Check sheet for the modelled part. Datum: model origin and axes. Units: mm. Face numbers are marked on the shaded views. Give positions to 0.01 mm unless a question says otherwise; leave off trailing zeros. Loops run counter-clockwise (first coordinate to the right, second up) from the corner with the lowest first, then second, coordinate; pieces in that order, holes last. Notation, with made-up numbers: (64, 12.25) - (85, 12.25) arc R18 ccw to (85, 42.25) - close; hole circle Ø9 at (29.25, 64.5). An arc over 180 degrees is marked (long way). Use CSV: the item, a comma, the result in double quotes.
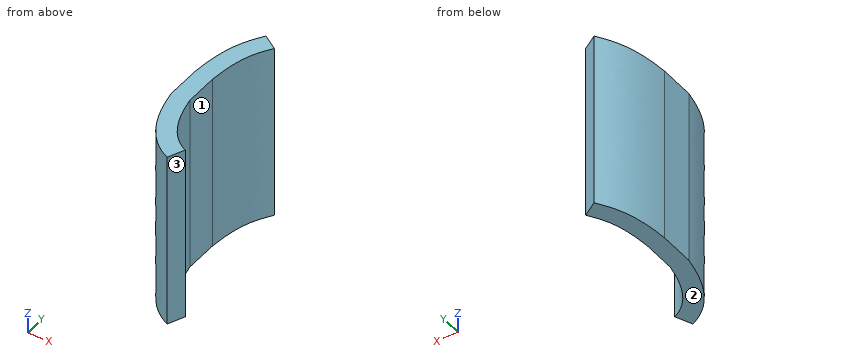
from build123d import *

# Parameters (mm, degrees)
BOSS_EXTRUDE1_DEPTH = 100


with BuildPart() as part:
    # Sketch2 → Boss-Extrude1 (new body)
    with BuildSketch(Plane.XY):
        with BuildLine():
            add(Edge.make_bspline(
                [(0, 10), (1.533515377, 33.319151282), (7.303166768, 41.847313143), (12.598069813, 50)],
                knots=[0, 0, 0, 0, 1, 1, 1, 1], degree=3))
            Line((0, 10), (0, 0))
            Line((0, 0), (0, -10))
            add(Edge.make_bspline(
                [(0, -10), (5.162408831, -41.387474282), (24.940857621, -50)],
                knots=[0, 0, 0, 1, 1, 1], degree=2))
            Line((24.940857621, -50), (28.933264328, -40.831538368))
            add(Edge.make_bspline(
                [(10, -9.163474156), (10.056385248, -9.489994067), (10.218691454, -10.40274145), (10.608632812, -12.423582905), (11.217159707, -15.147367418), (12.036197112, -18.205876092), (13.241421003, -22.010184853), (14.946624948, -26.249584187), (17.264049235, -30.529570228), (19.809393711, -34.048772515), (22.561889728, -36.886540275), (25.055614435, -38.769105307), (27.20346958, -40.024321521), (28.35268275, -40.578724115), (28.933264328, -40.831538368)],
                knots=[0.013914319, 0.013914319, 0.013914319, 0.013914319, 0.03125, 0.0625, 0.125, 0.1875, 0.25, 0.375, 0.5, 0.625, 0.75, 0.875, 0.9375, 1, 1, 1, 1], degree=3))
            Line((10, -9.163474156), (10, 0))
            Line((10, 0), (10, 9.66613227))
            add(Edge.make_bspline(
                [(10, 9.66613227), (10.044832415, 10.325668243), (10.145323413, 11.665207775), (10.370656318, 14.172612644), (10.703199446, 17.109625288), (11.171932341, 20.302311995), (11.878481202, 24.159772501), (12.891303178, 28.284538206), (14.25087497, 32.33124201), (15.719533079, 35.71915175), (17.301714969, 38.710204086), (18.75029356, 41.091588426), (19.993631129, 43.030159771), (20.657608588, 44.049863049), (20.984546989, 44.553257801)],
                knots=[0.004937345, 0.004937345, 0.004937345, 0.004937345, 0.036033053, 0.067128761, 0.129320177, 0.191511593, 0.253703009, 0.378085841, 0.502468673, 0.626851505, 0.751234336, 0.875617168, 0.937808584, 1, 1, 1, 1], degree=3))
            Line((20.984546989, 44.553257801), (12.598069813, 50))
        make_face()
    extrude(amount=BOSS_EXTRUDE1_DEPTH)


solid = part.part
1. Sectioned sample at A-A, the plane y = 3. Record the boundary of the cut face in (x, z), and give its area (3 significant figures).
Completed:
outline,"(0, 0) - (10, 0) - (10, 100) - (0, 100) - close"
area,"1,000 mm²"
2. Release check for a two-part mould opening along Y. For the marked faces 1, 2 and 3 record: released by +Y, released by -Y, zero draft, split by the parting line, or undercut.
Completed:
face 1,"undercut"
face 2,"zero draft"
face 3,"released by -Y"
3. Go/stop test with flat-tipped pins: pin 1 Ø6 at (x, z) = (19.5, 72) entering from -Y; pin 2 Ø1.5 at (x, z) = (8.5, 15.5) entering from +Y; pin 3 Ø6 at (x, y) = (21, -28.5) entering from -Z; pin 4 Ø4 at (y, z) = (-38.5, 21.5) entering from +X. Record where each tip stops, or that it passes through.
Completed:
pin 1,"stops at y = -48.82"
pin 2,"stops at y = 44.69"
pin 3,"passes through"
pin 4,"stops at x = 28.2"
4. Scan lines: line 1 along Y through (x, z) = (20.25, 66); line 2 along X through (y, z) = (-8, 16); line 3 along Y through (x, z) = (6.25, 16). Record each from-to range of solid material in increasing order.
Completed:
line 1,"y = -47.51 to -34.41, 43.42 to 45.03"
line 2,"x = 0 to 10"
line 3,"y = -31.02 to 38.97"
